from build123d import *

# Parameters (mm, degrees)
CHAMFER1_SIZE      = 1
CUT_EXTRUDE1_DEPTH = 10


with BuildPart() as part:
    # Sketch1 → Revolve1 (revolve)
    with BuildSketch(Plane.XY, mode=Mode.PRIVATE) as revolve1_sk:
        Polygon((0, 0), (0, 5), (-13, 5), (-13, 4), (-15, 4), (-15, 10), (-29, 10), (-29, 12.5), (-53, 12.5), (-53, 17), (-75, 17), (-75, 10), (-97, 10), (-97, 6.5), (-100, 6.5), (-100, 8), (-118, 8), (-118, 0), align=None)
    revolve(revolve1_sk.sketch.rotate(Axis((0, 0, 0), (-1, 0, 0)), 90), axis=Axis((0, 0, 0), (-1, 0, 0)))

    # Chamfer1
    chamfer1_edges = [part.edges().sort_by_distance(p)[0] for p in [
        (-118, 0, 8),
        (-97, 0, 10),
        (-53, 0, 17),
        (-29, 0, 12.5),
        (-15, 0, 10),
        (0, 0, 5),
    ]]
    chamfer(chamfer1_edges, length=CHAMFER1_SIZE)

    # Sketch2 → Cut-Extrude1 (cut)
    with BuildSketch(Plane.ZY.offset(75)):
        with BuildLine():
            Line((-14, -9.643650761), (-14, 9.643650761))
            ThreePointArc((-14, 9.643650761), (-17, 0), (-14, -9.643650761))
        make_face()
        with BuildLine():
            ThreePointArc((17, 0), (16.232683081, 5.049752469), (14, 9.643650761))
            Line((14, 9.643650761), (14, -9.643650761))
            ThreePointArc((14, -9.643650761), (16.232683081, -5.049752469), (17, 0))
        make_face()
    extrude(amount=-CUT_EXTRUDE1_DEPTH, mode=Mode.SUBTRACT)


solid = part.part
Part model, mm, in its own coordinate system. A direction names the side the tool comes from. Round coordinates to 2 decimals unless told otherwise and drop trailing zeros. Loops run counter-clockwise (first coordinate to the right, second up) from the corner with the lowest first, then second, coordinate; pieces in that order, holes last. Notation, with made-up numbers: (74, 31.25) - (103, 31.25) arc R32 cw to (103, 57.25) - close; hole circle Ø10 at (82, 40). An arc over 180 degrees is marked (long way). Answer as a JSON object with one key per item and string values.
Item 1: Wall check: L1, parallel to Z at x = -67, y = -8.5; L2, parallel to X at y = -13, z = 8; L3, parallel to X at y = 3, z = -8.5. Give the ranges that are in metal, low to high.
Output:
{"L1": "-14 to 14", "L2": "-75 to -53", "L3": "-96.99 to -15.01"}
Item 2: Pull direction X, two halves, no side cores. Call faces 5 (the face through (-75, 4, 10)), 6 (the face through (-100, -7, 0)), 7 (the face through (-29, -5, -9)), 8 (the face through (-70, 0, -14)): pulls with the +X half, pulls with the -X half, needs draft (parallel to the pull), parting line crosses it, or undercut.
Output:
{"face 5": "pulls with the -X half", "face 6": "undercut", "face 7": "pulls with the +X half", "face 8": "needs draft"}
Item 3: Band-saw the part on B-B on x = -83. List the corners of the cut face in (y, z), plus the area to 3 significant figures.
Output:
{"outline": "circle Ø20 at (0, 0)", "area": "314 mm2"}
Item 4: Band-saw the part on A-A on x = -107. List the corners of the cut face in (y, z), plus the area to 3 significant figures.
Output:
{"outline": "circle Ø16 at (0, 0)", "area": "201 mm2"}
Item 5: Pin check, flat tips, straight feed: pin 1 (8 mm diameter, centred on x = -71.5, y = 4.5, fed in from +Z); pin 2 (8 mm diameter, centred on x = -58, y = 6.5, fed in from -Z); pin 3 (10 mm diameter, centred on x = -49.5, y = 3.5, fed in from +Z); pin 4 (2 mm diameter, centred on x = -101.5, z = 10.5, fed in from -Y). Stop position of each tip, or through.
Output:
{"pin 1": "z = 14", "pin 2": "z = -16.82", "pin 3": "z = 16.95", "pin 4": "through"}
Item 6: Tool access for faces 1 (the face through (-86, 0, 10)), 2 (the face through (-97, 6, -3)), 3 (the face through (-41.661, -3.755, -11.923)), 4 (the face through (-70, 0, 14)): list every direction of +Z, -Z, +X, -X, +Y, -Y with a clear straight run to the whole face (end or side of a thin tool).
Output:
{"face 1": "-X", "face 2": "none", "face 3": "+X", "face 4": "+Z, -X, +Y, -Y"}
